Autodesk Fusion 360 part; units mm, degrees
sketch "Skizze3" plane through (0, 0, 0) normal (0, 1, 0) x (1, 0, 0)
  line L0 (0, 0) -> (0, 13)
  line L1 (0, 13) -> (8, 13)
  line L2 (8, 13) -> (8, 11)
  line L3 (8, 11) -> (7.5, 11)
  line L4 (7.5, 11) -> (7.5, 0)
  line L5 (1.75, 0) -> (22.5, 0)
  line L6 (0, 0) -> (0, -13)
  line L7 (0, -13) -> (8, -13)
  line L8 (8, -11) -> (7.5, -11)
  line L9 (7.5, -11) -> (7.5, 0)
  line L10 (8, -13) -> (8, -11)
  dimension "d14" = 13
  dimension "d15" = 8
  dimension "d16" = 2
  dimension "d17" = 0.5
revolve "Drehen1" add sketch "Skizze3" angle 360 about axis through (0, 0, 0) along (0, 0, 1)
hole "Bohrung1" at (0, 0, 13) direction (0, 0, -1) diameter 12.5 end through all
ref_plane "Arbeitsebene1" through (0, 7.5, 0) normal (0, 1, 0) x (0, 0, 1)
sketch "Skizze5" plane through (0, 7.5, 0) normal (0, 1, 0) x (1, 0, 0)
  circle A0 centre (0, 8.3) radius 1
  dimension "d24" = 2
extrude "Extrusion3" cut sketch "Skizze5" against normal blind 3
component "Component" placed x (1, 0, 0) y (0, 1, 0) z (0, 0, 1) at (0, 0, 0)
Work out the finished part from the listing and answer in its coordinate system (mm). A direction names the side the tool comes from. Round coordinates to 2 decimals unless told otherwise and drop trailing zeros. Loops run counter-clockwise (first coordinate to the right, second up) from the corner with the lowest first, then second, coordinate; pieces in that order, holes last. Notation, with made-up numbers: M -12.75,18 L 36.25,18 A13 ccw 36.25,22 Z; hole C 44,-21.5 d5. An arc over 180 degrees is marked long. One line per question, with ' | ' between items. Start each with the question number.
(1) A cutting plane is placed at A-A on y = 0. Write down the section's boundary in (x, z), plus the area to 3 significant figures.
(2) Flat-ended cylindrical pins translate along their axes: pin 1 Ø1.5 at (x, z) = (4, 7.5) entering from +Y; pin 2 Ø1.2 at (x, z) = (0, -8.3) entering from -Y; pin 3 Ø3 at (y, z) = (0.5, -2.5) entering from +X. Find the tip coordinate at first contact, or state that the pin passes through.
(3) A cutting plane is placed at B-B on x = 3.75. Write down the section's boundary in (y, z).
(4) A cutting plane is placed at C-C on z = 2. Write down the section's boundary in (x, y).
(5) A tool of negligible diameter and unlimited length cuts with its end or side. For faces 5 (the face through (-5, -4, 13)), 6 (the face through (-7.493, 0.33, 0.154)), from which of +Z, -Z, +X, -X, +Y, -Y can it reach the whole face along a straight path? Write none if from no direction.
(6) For a pull along Z with two mould halves and no side action, classify faces 1 (the face through (-5, -4, -13)), 2 (the face through (-1.73, 7.81, 11.99)), 3 (the face through (0.954, 6.844, -8.6)), 4 (the face through (5, -6, -11)) as released by +Z, released by -Z, zero draft, split by the parting line, or undercut.
(7) Find the intervals of material crossed by line 1 (Y direction, x = 0, z = -4.5); line 2 (Z direction, x = 0, y = 6.5); line 3 (Y direction, x = -2.75, z = 2), in increasing order.
(8) A cutting plane is placed at D-D on y = 7. Write down the section's boundary in (x, z), plus the area to 3 significant figures.
Geometry check:
1) outline: M -8,-13 L -6.25,-13 L -6.25,13 L -8,13 L -8,11 L -7.5,11 L -7.5,-11 L -8,-11 Z; M 6.25,-13 L 8,-13 L 8,-11 L 7.5,-11 L 7.5,11 L 8,11 L 8,13 L 6.25,13 Z | area: 69.0 mm²
2) pin 1: stops at y = 6.76 | pin 2: stops at y = -7.5 | pin 3: stops at x = 7.5
3) outline: M -7.07,-13 L -5,-13 L -5,13 L -7.07,13 L -7.07,11 L -6.5,11 L -6.5,-11 L -7.07,-11 Z; M 5,-13 L 7.07,-13 L 7.07,-11 L 6.5,-11 L 6.5,11 L 7.07,11 L 7.07,13 L 5,13 Z
4) outline: C 0,0 d15; hole C 0,0 d12.5
5) face 5: +Z, +X, -X, +Y, -Y | face 6: none
6) face 1: released by -Z | face 2: zero draft | face 3: undercut | face 4: undercut
7) line 1: y = -7.5 to -6.25, 6.25 to 7.5 | line 2: z = -13 to -9.3, -7.3 to 13 | line 3: y = -6.98 to -5.61, 5.61 to 6.98
8) outline: M -3.87,-13 L 3.87,-13 L 3.87,-11 L 2.69,-11 L 2.69,11 L 3.87,11 L 3.87,13 L -3.87,13 L -3.87,11 L -2.69,11 L -2.69,-11 L -3.87,-11 Z; hole C 0,-8.3 d2 | area: 146 mm²
